from build123d import *

# Parameters (mm, degrees)
EXTRUDE_1_DEPTH = 14.5
FILLET_1_R      = 3
FILLET_2_R      = 0.5


with BuildPart() as part:
    # 草图1 → 凸台-拉伸1 (new body)
    with BuildSketch(Plane(origin=(0, 0, 0), x_dir=(1, 0, 0), z_dir=(0, 1, 0))):
        Polygon((0, 0), (6.5, 4), (6.5, -15), (11.5, -15), (11.5, -20), (-5, -20), (-5, -15), (0, -15), align=None)
    extrude(amount=EXTRUDE_1_DEPTH)

    # 圆角1
    fillet_1_edges = [part.edges().sort_by_distance(p)[0] for p in [
        (0, 7.25, 0),
    ]]
    fillet(fillet_1_edges, radius=FILLET_1_R)

    # 圆角2
    fillet_2_edges = [part.edges().sort_by_distance(p)[0] for p in [
        (6.5, 7.25, -4),
    ]]
    fillet(fillet_2_edges, radius=FILLET_2_R)


solid = part.part
Could you check a few things on this model? Use its own coordinates, in mm. A direction names the side the tool comes from. Give positions to 0.01 mm unless a question says otherwise; leave off trailing zeros. Loops run counter-clockwise (first coordinate to the right, second up) from the corner with the lowest first, then second, coordinate; pieces in that order, holes last. Notation, with made-up numbers: M -7.75,63 L 19.25,63 A21 ccw 19.25,68 Z; hole C 26,34.25 d7. An arc over 180 degrees is marked long. Answer as a JSON object with one key per item and string values.
Q1. If I drill on probe 1 along Z at (x, y) = (-1.5, 12.5); probe 2 along X at (y, z) = (3.75, 2.5); probe 3 along X at (y, z) = (9, 1), over which ranges is the centre line in solid material (lowest first)? Write a range as [from, to].
Values found:
{"probe 1": "z = [15, 20]", "probe 2": "x = [0, 6.5]", "probe 3": "x = [0.08, 6.5]"}
Q2. Suppose I cut it at A-A, the plane y = 6. List the corners of the cut face in (x, z) for me, plus the area to 3 significant figures.
Values found:
{"outline": "M -5,15 L 0,15 L 0,1.68 A3 ccw 1.43,-0.88 L 5.74,-3.53 A0.5 ccw 6.5,-3.11 L 6.5,15 L 11.5,15 L 11.5,20 L -5,20 Z", "area": "192 mm²"}
Q3. For faces 1 (the flat face through (9, 7, 15)), 2 (the flat face through (3, 0, 11)), 3 (the flat face through (-3, 7, 15)), which set-ups out of +Z, -Z, +X, -X, +Y, -Y let a thin tool reach every point of the face, with its end or its side?
Values found:
{"face 1": "-Z, +X, +Y, -Y", "face 2": "+Z, -Z, +X, -X, -Y", "face 3": "-Z, -X, +Y, -Y"}
Q4. Suppose I cut it at B-B, the plane z = 8.75. List the corners of the cut face in (x, y) for me, plus the area to 4 significant figures.
Values found:
{"outline": "M 0,0 L 6.5,0 L 6.5,14.5 L 0,14.5 Z", "area": "94.25 mm²"}
Q5. Suppose I cut it at C-C, the plane x = -2. List the corners of the cut face in (y, z) for me, plus the area to 3 significant figures.
Values found:
{"outline": "M 0,15 L 14.5,15 L 14.5,20 L 0,20 Z", "area": "72.5 mm²"}
Q6. For P1, Ø2, axis at x = 2, y = 9.5, coming from the -Z side; P2, Ø1.5, axis at y = 6, z = 10.5, coming from the -X side; P3, Ø2.5, axis at x = -3, y = 10.5, coming from the -Z side; P4, Ø4, axis at x = -3, z = -1, coming from the -Y side, each with a flat end and sliding along its axis, tell me the tip position at first contact or that it passes through.
Values found:
{"P1": "stops at z = -1.85", "P2": "stops at x = 0", "P3": "stops at z = 15", "P4": "passes through"}
